from build123d import *

# Parameters (mm, degrees)
F1_DEPTH = 2.5
F0_W     = 1
F0_H     = 0.75
F2_DEPTH = 1.5
F3_DEPTH = 1


with BuildPart() as f1:
    # F0 (on Front) → F1 (new body, symmetric)
    with BuildSketch(Plane.XZ):
        Polygon((1.625, -0.375), (1.625, 0.375), (0.875, 0.375), (-1.625, 0.375), (-1.625, -0.375), align=None)
    extrude(amount=F1_DEPTH, both=True)

    # F0 (on Front) → F2 (join, symmetric)
    with BuildSketch(Plane.XZ):
        with BuildLine():
            Line((0.875, 0.375), (1.625, 0.375))
            Line((1.625, 0.375), (1.625, 1.063))
            ThreePointArc((1.625, 1.063), (1.8080582618, 1.5049417382), (2.25, 1.688))
            Line((2.25, 1.688), (2.375, 1.688))
            Line((2.375, 1.688), (2.375, 2.438))
            Line((2.375, 2.438), (2.25, 2.438))
            add(Edge.make_bspline(
                [(2.170906051, 2.4357232595), (2.1971042738, 2.4365893648), (2.2234685803, 2.4373486386), (2.25, 2.438)],
                knots=[4.3419944686, 4.3419944686, 4.3419944686, 4.3419944686, 4.3899423686, 4.3899423686, 4.3899423686, 4.3899423686], degree=3))
            ThreePointArc((2.170906051, 2.4357232595), (1.2501552171, 2.0068937493), (0.875, 1.063))
            Line((0.875, 1.063), (0.875, 0.375))
        make_face()
        with Locations((2.875, 2.063)):
            Rectangle(F0_W, F0_H)
    extrude(amount=F2_DEPTH, both=True)

    # F0 (on Front) → F3 (join, symmetric)
    with BuildSketch(Plane.XZ):
        with BuildLine():
            Line((-1.625, 0.375), (0.875, 0.375))
            Line((0.875, 0.375), (0.875, 1.063))
            ThreePointArc((0.875, 1.063), (1.2501552171, 2.0068937493), (2.170906051, 2.4357232595))
            add(Edge.make_bspline(
                [(-1.625, 0.375), (-1.2119672171, 1.4027909671), (-0.2015135657, 2.3572917876), (2.170906051, 2.4357232595)],
                knots=[0, 0, 0, 0, 4.3419944686, 4.3419944686, 4.3419944686, 4.3419944686], degree=3))
        make_face()
    extrude(amount=F3_DEPTH, both=True)

    # F0 (on Front) → F4 (revolve)
    with BuildSketch(Plane.XZ):
        Polygon((3.375, 2.438), (3.375, 1.688), (3.375, 1.5), (4.375, 1.5), (4.375, 2.625), (3.375, 2.625), align=None)
    revolve(axis=Axis((3.375, 0, 2.0625), (0, 0, 1)))


solid = f1.part
Here's how the part is built. I have some questions about the finished solid (model axes, mm). A direction names the side the tool comes from. Coordinates: 2 decimals unless noted, no trailing zeros. Loops run counter-clockwise (first coordinate to the right, second up) from the corner with the lowest first, then second, coordinate; pieces in that order, holes last. Notation, with made-up numbers: (-2.5, 71.25) -> (28.5, 71.25) arc R23 cw to (28.5, 107.25) -> close; hole circle Ø10 at (28.25, -14). An arc over 180 degrees is marked (long way). Use one line per item in the form item = value. Start each with the question number.
(1) If we section it at C-C (x = 4.25): Please give me the cut outline in (y, z) (3 decimals).
(2) We'd pull the mould along X, two halves only. Please class faces 5 (the face through (1.625, 0, 0)), 6 (the face through (2.43, -0.69, 1.688)), 7 (the face through (1.26, 1.25, 2.02)), 8 (the face through (0, -2, 0.375)): pulls with the +X half, pulls with the -X half, needs draft (parallel to the pull), parting line crosses it, or undercut.
(3) On a 3-axis mill with a long thin cutter (end or side, diameter ignored), from which of +Z, -Z, +X, -X, +Y, -Y can I reach the whole of each face in a straight line? I mean faces 1 (the face through (2, 1.5, 2)), 2 (the face through (0, -1, 1)), 3 (the face through (0, 1, 1)), 4 (the face through (2, -1.5, 2)). Say none if no direction works.
(4) If we section it at B-B (y = 2): Please give me the cut outline in (x, z) (3 decimals), then the cut area to 3 significant figures.
(5) Will these pins go through, and if not, where does the flat tip stop? pin 1 (1.2 mm diameter, centred on x = -0.5, y = -2, fed in from +Z) (3 decimals); pin 2 (1 mm diameter, centred on x = 2, z = 2, fed in from -Y); pin 3 (0.6 mm diameter, centred on x = 2.5, y = 0.5, fed in from -Z); pin 4 (0.6 mm diameter, centred on x = 2, z = 1, fed in from +Y).
(6) Please list where these lines run through material, in increasing order: line 1 along Z through (x, y) = (4, -0.25) (3 decimals); line 2 along X through (y, z) = (-1.1, -0.05) (3 decimals); line 3 along X through (y, z) = (1.1, 0.75) (3 decimals).
(7) If we section it at A-A (x = 3.25): Please give me the cut outline in (y, z) (3 decimals).
Verdict:
q1.outline = (-0.484, 1.5) -> (0.484, 1.5) -> (0.484, 2.625) -> (-0.484, 2.625) -> close
q2.face_5 = pulls with the +X half
q2.face_6 = undercut
q2.face_7 = pulls with the -X half
q2.face_8 = needs draft
q3.face_1 = +Z, +X, -X, +Y
q3.face_2 = +Z, -X, -Y
q3.face_3 = +Z, -X, +Y
q3.face_4 = +Z, +X, -X, -Y
q4.outline = (-1.625, -0.375) -> (1.625, -0.375) -> (1.625, 0.375) -> (-1.625, 0.375) -> close
q4.area = 2.44 mm²
q5.pin_1 = 0.375
q5.pin_2 = -1.5
q5.pin_3 = 1.5
q5.pin_4 = through
q6.line_1 = 1.5 to 2.625
q6.line_2 = -1.625 to 1.625
q6.line_3 = 0.875 to 1.625
q7.outline = (-1.5, 1.688) -> (-0.992, 1.688) -> (-0.992, 1.5) -> (0.992, 1.5) -> (0.992, 1.688) -> (1.5, 1.688) -> (1.5, 2.438) -> (0.992, 2.438) -> (0.992, 2.625) -> (-0.992, 2.625) -> (-0.992, 2.438) -> (-1.5, 2.438) -> close
